```python
from build123d import *

# Parameters (mm, degrees)
F0_W     = 60
F0_H     = 60
F1_DEPTH = 20
F2_W     = 60
F2_H     = 20
F3_DEPTH = 40
F5_DEPTH = 25


with BuildPart() as f1:
    # F0 (on Top) → F1 (new body)
    with BuildSketch(Plane.XY):
        with Locations((30, 30)):
            Rectangle(F0_W, F0_H)
    extrude(amount=-F1_DEPTH)

    # F2 (on face) → F3 (join)
    with BuildSketch(Plane(origin=(0, 0, -20), x_dir=(1, 0, 0), z_dir=(0, 0, -1))):
        with Locations((30, -50)):
            Rectangle(F2_W, F2_H)
    extrude(amount=-F3_DEPTH)

    # F4 (on face) → F5 (cut)
    with BuildSketch(Plane.XZ.offset(-40)):
        with BuildLine():
            Line((45, 20), (15, 20))
            ThreePointArc((15, 20), (30, 5), (45, 20))
        make_face()
    extrude(amount=-F5_DEPTH, mode=Mode.SUBTRACT)


solid = f1.part
```
Model file for the job. Use its own axes, mm. A direction names the side the tool comes from. Round coordinates to 2 decimals unless told otherwise and drop trailing zeros. Write each loop counter-clockwise with the first axis right and the second up, starting at its lowest first coordinate (ties: lowest second). Pieces come first, ordered by that corner, then holes. Notation, with made-up numbers: (21, 57.5) - (74, 57.5) arc R13 cw to (74, 77.5) - close; hole circle Ø8 at (60.25, -27). An arc over 180 degrees is marked (long way). Use CSV: the item, a comma, the result in double quotes. Start each with the question number.
Item 1: Drill centre lines: L1, parallel to Z at x = 44, y = 7; L2, parallel to X at y = 52.5, z = 11.5; L3, parallel to Y at x = 43, z = 7. Where is each one in solid material? Low to high. Write a range as [from, to].
Item 2: Two-plate mould, pull along X, no slides. Class faces 1 (the face through (30, 50, 5)), 2 (the face through (52, 50, 20)), 3 (the face through (0, 37, -5)): released by +X, released by -X, zero draft, split by the parting line, or undercut.
Item 3: Band-saw the part on D-D (z = 2.5). Write the cut outline in (x, y), and give its area (3 significant figures).
Item 4: Pin check, flat tips, straight feed: P1, Ø2, axis at x = 23, z = 9, coming from the +Y side; P2, Ø3, axis at x = 14.5, z = 10.5, coming from the -Y side; P3, Ø1.5, axis at x = 24, y = 33, coming from the +Z side. Stop position of each tip, or through.
Item 5: Band-saw the part on B-B (z = 13.5). Write the cut outline in (x, y), and give its area (3 significant figures).
Item 6: Tool access for faces 4 (the face through (30, 60, -5)), 5 (the face through (30, 20, 0)): list every direction of +Z, -Z, +X, -X, +Y, -Y with a clear straight run to the whole face (end or side of a thin tool).
Item 7: Band-saw the part on C-C (y = 39). Write the cut outline in (x, z), and give its area (3 significant figures).
Item 8: Band-saw the part on A-A (x = 30). Write the cut outline in (y, z).
Checked values:
1,L1,"z = [-20, 0]"
1,L2,"x = [0, 17.64], [42.36, 60]"
1,L3,"y = [40, 60]"
2,face 1,"undercut"
2,face 2,"zero draft"
2,face 3,"released by -X"
3,outline,"(0, 40) - (60, 40) - (60, 60) - (0, 60) - close"
3,area,"1,200 mm²"
4,P1,"passes through"
4,P2,"stops at y = 40"
4,P3,"stops at z = 0"
5,outline,"(0, 40) - (16.48, 40) - (16.48, 60) - (0, 60) - close; (43.52, 40) - (60, 40) - (60, 60) - (43.52, 60) - close"
5,area,"659 mm²"
6,face 4,"+Z, -Z, +X, -X, +Y"
6,face 5,"+Z, +X, -X, -Y"
7,outline,"(0, -20) - (60, -20) - (60, 0) - (0, 0) - close"
7,area,"1,200 mm²"
8,outline,"(0, -20) - (60, -20) - (60, 5) - (40, 5) - (40, 0) - (0, 0) - close"
